Part model, mm, in its own coordinate system. Face numbers are marked on the shaded views. A direction names the side the tool comes from. Coordinates: 2 decimals unless noted, no trailing zeros. Order: outer loops, then holes, each group sorted by start corner. A loop starts at its lowest first (then second) coordinate and runs counter-clockwise, first axis right, second up.
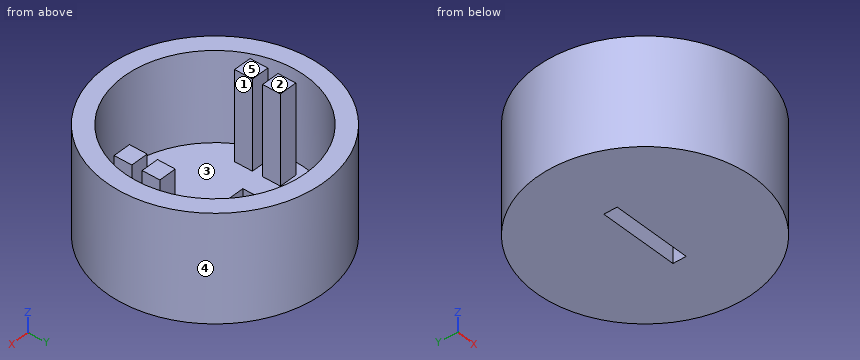
Autodesk Inventor part; units mm, degrees
ref_plane "YZ Plane" through (0, 0, 0) normal (1, 0, 0) x (0, 1, 0)
ref_plane "XZ Plane" through (0, 0, 0) normal (0, 1, 0) x (-1, 0, 0)
ref_plane "XY Plane" through (0, 0, 0) normal (0, 0, 1) x (1, 0, 0)
sketch "Sketch1" plane through (0, 0, 0) normal (0, 0, 1) x (1, 0, 0)
  circle A0 centre (0, 0) radius 12.25
  point P0 (0, 0)
extrude "Extrusion1" add sketch "Sketch1" along normal blind 2
sketch "Sketch2" plane through (0, 0, 2) normal (0, 0, 1) x (1, 0, 0)
  circle A0 centre (0, 0) radius 12.25
  line L0 (-4.5, -0.75) -> (4.5, -0.75)
  line L1 (4.5, -0.75) -> (4.5, 0.75)
  line L2 (4.5, 0.75) -> (-4.5, 0.75)
  line L3 (-4.5, 0.75) -> (-4.5, -0.75)
  line L4 (-4.5, -0.75) -> (4.5, 0.75) construction
  line L5 (4.5, -0.75) -> (-4.5, 0.75) construction
  dimension "d13" = 9
  dimension "d14" = 1.5
extrude "Extrusion2" cut sketch "Sketch2" against normal through all contours L3 L2 L1 L0
sketch "Sketch3" plane through (0, 0, 2) normal (0, 0, 1) x (1, 0, 0)
  circle A0 centre (0, 0) radius 12.25
  circle A1 centre (0, 0) radius 10.25
  dimension "d4" = 2
extrude "Extrusion3" add sketch "Sketch3" along normal blind 10
sketch "Sketch4" plane through (0, 0, 2) normal (0, 0, 1) x (1, 0, 0)
  circle A0 centre (0, 0) radius 10.25 construction
  line L0 (-5.235, -0.75) -> (-8.355, -0.75) construction
  line L1 (-5.235, -1.51) -> (-8.355, -1.51) construction
  line L2 (-8.355, -0.75) -> (-8.355, -1.51)
  line L3 (-8.855, -0.55) -> (-6.855, -0.55)
  line L4 (-6.855, -0.55) -> (-6.855, 1.45)
  line L5 (-6.855, 1.45) -> (-8.855, 1.45)
  line L6 (-8.855, 1.45) -> (-8.855, -0.55)
  line L7 (-8.855, -0.55) -> (-6.855, 1.45) construction
  line L8 (-6.855, -0.55) -> (-8.855, 1.45) construction
  line L9 (-8.355, -1.13) -> (-6.0393, -1.13) construction
  line L10 (-8.855, -1.71) -> (-6.855, -1.71)
  line L11 (-6.855, -1.71) -> (-6.855, -3.71)
  line L12 (-6.855, -3.71) -> (-8.855, -3.71)
  line L13 (-8.855, -3.71) -> (-8.855, -1.71)
  line L14 (-8.855, -1.71) -> (-6.855, -3.71) construction
  line L15 (-6.855, -1.71) -> (-8.855, -3.71) construction
  line L16 (0, 0) -> (0, -2.4826) construction
  line L17 (8.855, -0.55) -> (6.855, -0.55)
  line L18 (6.855, -0.55) -> (6.855, 1.45)
  line L19 (6.855, 1.45) -> (8.855, 1.45)
  line L20 (8.855, 1.45) -> (8.855, -0.55)
  line L21 (8.855, -0.55) -> (6.855, 1.45) construction
  line L22 (6.855, -0.55) -> (8.855, 1.45) construction
  line L23 (6.855, -1.71) -> (6.855, -3.71)
  line L24 (8.855, -1.71) -> (6.855, -1.71)
  line L25 (6.855, -3.71) -> (8.855, -3.71)
  line L26 (8.855, -1.71) -> (6.855, -3.71) construction
  line L27 (6.855, -1.71) -> (8.855, -3.71) construction
  line L28 (8.855, -3.71) -> (8.855, -1.71)
  point P0 (-7.855, 0.45)
  point P1 (-7.855, -2.71)
  point P2 (7.855, 0.45)
  point P3 (7.855, -2.71)
  dimension "d7" = 0.2
  dimension "d8" = 0.5
  dimension "d9" = 2
  dimension "d10" = 2
extrude "Extrusion4" add sketch "Sketch4" along normal up to surface (10 mm away)
properties part number "PI_holder"
(1) Drop flat-ended pins along their axis: pin 1 (1 mm diameter, centred on x = 8, z = 7, fed in from -Y); pin 2 (2 mm diameter, centred on x = -8, z = 8.5, fed in from -Y); pin 3 (1 mm diameter, centred on y = 8, z = 8.5, fed in from +X). Give the stop position or say it passes through.
(2) Tool access for the marked faces 1 and 2: list every direction of +Z, -Z, +X, -X, +Y, -Y with a clear straight run to the whole face (end or side of a thin tool).
(3) Slice it at D-D, the plane y = -6.25. Give the cut face in (x, z).
(4) Pull direction Y, two halves, no side cores. Call the marked faces 3, 4 and 5: +Y half, -Y half, draft (parallel to the pull), parting line (faces both ways), or undercut.
(5) Probe line 1 (Y direction, x = 0, z = 7.5); line 2 (Y direction, x = -8.5, z = 6.5); line 3 (Y direction, x = -7, z = 9.5). List the from-to ranges inside material, lowest first.
(6) Slice it at C-C, the plane x = 0. Give the cut face in (y, z), then the cut area to 3 significant figures.
(7) Slice it at B-B, the plane y = 0. Give the cut face in (x, z) (3 decimals).
(8) Slice it at A-A, the plane z = 4.75. Give the cut face in (x, y) (3 decimals).
Here are the results:
1. pin 1: stops at y = -9.69
1. pin 2: stops at y = -10.05
1. pin 3: stops at x = 9.69
2. face 1: +Z
2. face 2: +Z, +X, -X, +Y, -Y
3. outline: (-10.54, 0) - (10.54, 0) - (10.54, 12) - (8.12, 12) - (8.12, 2) - (-8.12, 2) - (-8.12, 12) - (-10.54, 12) - close
4. face 3: undercut
4. face 4: parting line
4. face 5: draft
5. line 1: y = -12.25 to -10.25, 10.25 to 12.25
5. line 2: y = -8.82 to -5.73, -3.71 to -1.71, -0.55 to 1.45, 5.73 to 8.82
5. line 3: y = -10.05 to -7.49, -3.71 to -1.71, -0.55 to 1.45, 7.49 to 10.05
6. outline: (-12.25, 0) - (-0.75, 0) - (-0.75, 2) - (-10.25, 2) - (-10.25, 12) - (-12.25, 12) - close; (0.75, 0) - (12.25, 0) - (12.25, 12) - (10.25, 12) - (10.25, 2) - (0.75, 2) - close
6. area: 86.0 mm2
7. outline: (-12.25, 0) - (-4.5, 0) - (-4.5, 2) - (-6.855, 2) - (-6.855, 12) - (-8.855, 12) - (-8.855, 2) - (-10.25, 2) - (-10.25, 12) - (-12.25, 12) - close; (4.5, 0) - (12.25, 0) - (12.25, 12) - (10.25, 12) - (10.25, 2) - (8.855, 2) - (8.855, 12) - (6.855, 12) - (6.855, 2) - (4.5, 2) - close
8. outline: circle Ø24.5 at (0, 0); (-8.855, -3.71) - (-6.855, -3.71) - (-6.855, -1.71) - (-8.855, -1.71) - close; (-8.855, -0.55) - (-6.855, -0.55) - (-6.855, 1.45) - (-8.855, 1.45) - close; (6.855, -3.71) - (8.855, -3.71) - (8.855, -1.71) - (6.855, -1.71) - close; (6.855, -0.55) - (8.855, -0.55) - (8.855, 1.45) - (6.855, 1.45) - close; hole circle Ø20.5 at (0, 0)
